Autodesk Inventor part; units mm, degrees
ref_plane "YZ Plane" through (0, 0, 0) normal (1, 0, 0) x (0, 1, 0)
ref_plane "XZ Plane" through (0, 0, 0) normal (0, 1, 0) x (-1, 0, 0)
ref_plane "XY Plane" through (0, 0, 0) normal (0, 0, 1) x (1, 0, 0)
sketch "Эскиз1" plane through (0, 0, 0) normal (0, 1, 0) x (-1, 0, 0)
  line L0 (0, 0) -> (-200, 0)
  line L1 (-200, 0) -> (-200, -30)
  line L2 (-200, -30) -> (0, -30)
  line L3 (0, -30) -> (0, 0)
  dimension "d0" = 200
  dimension "d1" = 30
extrude "Выдавливание1" add sketch "Эскиз1" along normal blind 80
chamfer "Фаска1" distance 30 angle 45 2 edges at (0, 40, 0) (200, 40, 0)
sketch "Эскиз2" plane through (30, 0, 0) normal (0, 0, 1) x (1, 0, 0)
  line L0 (60, 55) -> (80, 55)
  line L1 (80, 55) -> (80, 25)
  line L2 (80, 25) -> (60, 25)
  line L3 (60, 25) -> (60, 55)
  line L4 (0, 0) -> (0, 80)
  line L5 (0, 80) -> (140, 80)
  point P0 (-30, 0)
  point P1 (60, 40)
  point P2 (0, 40)
  point P3 (70, 55)
  point P4 (70, 80)
  dimension "d7" = 20
  dimension "d8" = 30
extrude "Выдавливание2" cut sketch "Эскиз2" against normal through all
sketch "Эскиз3" plane through (0, 80, 0) normal (0, 1, 0) x (1, 0, 0)
  line L0 (200, 30) -> (170, 0)
  line L1 (200, 30) -> (0, 30)
  line L2 (30, 0) -> (0, 30)
  line L3 (30, 0) -> (170, 0)
  line L4 (30, 0) -> (0, 30)
  line L5 (15, 15) -> (7.9289, 22.0711)
  arc A0 (192.0711, 22.0711) -> (7.9289, 22.0711) centre (100, -508.5309) ccw
  line L6 (200, 30) -> (0, 30)
  line L7 (30, 0) -> (170, 0)
  arc A1 (170, 0) -> (30, 0) centre (100, -508.5309) ccw
  point P0 (0, 0)
  point P1 (100, 0)
  point P2 (100, 0)
  dimension "d11" = 10
extrude "Выдавливание3" cut sketch "Эскиз3" against normal through all contours L0 A0 L1 | A0 L2 L1 | L3 A1
sketch "Эскиз4" plane through (192.0711, 0, -22.0711) normal (0.7071068, 0, 0.7071068) x (0.7071068, 0, -0.7071068)
  line L0 (0, 0) -> (0, 80)
  line L1 (0, 80) -> (-31.2132, 80)
  line L2 (-31.2132, 80) -> (-31.2132, 0)
  line L3 (-31.2132, 0) -> (0, 0)
  line L4 (0, 80) -> (-130.2082, 80)
  arc A0 (-11.2132, 0) -> (-11.2132, 80) centre (-76.9511, 40) ccw
  arc A1 (-31.2132, 0) -> (-31.2132, 80) centre (-76.9511, 40) ccw
  line L5 (-31.2132, 0) -> (0, 0)
  line L6 (0, 0) -> (0, 80)
  line L7 (-31.2132, 80) -> (-11.2132, 80)
  line L8 (-31.2132, 0) -> (-11.2132, 0)
  point P0 (-151.4214, 0)
  point P1 (-31.2132, 40)
  dimension "d14" = 20
sketch3d "3D эскиз1"
  arc A0 (192.0711, 80, -22.0711) -> (7.9289, 80, -22.0711) centre (100, 80, 508.5309) ccw
sweep "Сдвиг1" cut profiles "Эскиз4" path "3D эскиз1" contours L3 A0 L0 | A0 L1 L0 | L2 A1
properties part number "dou_short_square" material "Красное дерево"
Build history of the part. All positions in model axes, mm. A direction names the side the tool comes from. Give positions to 0.01 mm unless a question says otherwise; leave off trailing zeros. Put each result on its own line as item: value.
Item 1: Wall check: probe 1 along X at (y, z) = (54.5, -15.5); probe 2 along Y at (x, z) = (155.5, -2.25); probe 3 along Y at (x, z) = (167, -6.75). Give the ranges that are in metal, low to high.
Results are:
probe 1: 14.5 to 90, 110 to 185.5
probe 2: 0 to 0.67, 79.33 to 80
probe 3: 0 to 11.39, 68.61 to 80
Item 2: Which spindle directions (+Z, -Z, +X, -X, +Y, -Y) get a long thin tool onto all of the face, cutting with end or side? Do faces 4 (the face through (110, 40, -22)), 5 (the face through (183, 39, -13)). Say none if no direction does.
Results are:
face 4: +Z, -Z
face 5: +Z, +X, +Y, -Y
Item 3: Pull direction Y, two halves, no side cores. Call faces 1 (the face through (101, 0, -13)), 2 (the face through (100, 25, -22)), 3 (the face through (101, 80, -13)): +Y half, -Y half, draft (parallel to the pull), parting line (faces both ways), or undercut.
Results are:
face 1: -Y half
face 2: undercut
face 3: +Y half
Item 4: Drop flat-ended pins along their axis: pin 1 Ø10 at (x, y) = (147.5, 23) entering from +Z; pin 2 Ø3 at (y, z) = (71, -18) entering from -X; pin 3 Ø2 at (x, y) = (86, 62.5) entering from +Z. Give the stop position or say it passes through.
Results are:
pin 1: z = -11.29
pin 2: x = 12.09
pin 3: z = -12.85
